Read the model definition and answer for the solid it produces. Units are mm, in the model's axes. Face numbers are marked on the shaded views. A direction names the side the tool comes from. Coordinates: 2 decimals unless noted, no trailing zeros. Order: outer loops, then holes, each group sorted by start corner. A loop starts at its lowest first (then second) coordinate and runs counter-clockwise, first axis right, second up. Notation, with made-up numbers: M 35.25,31.5 L 64.25,31.5 A13 ccw 64.25,43.5 Z; hole C 5.5,62.25 d5. An arc over 180 degrees is marked long. Put each result on its own line as item: value.
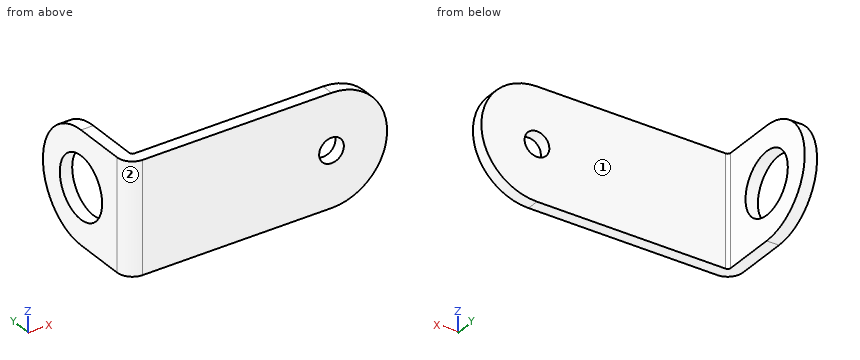
from build123d import *

# Parameters (mm, degrees)
BASE_FLANGE1_DEPTH = 14.2875
SKETCH8_R          = 7.9375
CUT_EXTRUDE3_DEPTH = 72.083846838
SKETCH7_R          = 3.175
CUT_EXTRUDE2_DEPTH = 72.083846838
FILLET1_RADIUS     = 14.2875
FILLET1_LENGTH     = 3.175
FILLET2_RADIUS     = 14.2875
FILLET2_LENGTH     = 3.175


# Sheet-metal steps are written as plain solids
with BuildPart() as part:
    # Sketch1 → Base-Flange1 (new, symmetric)
    with BuildSketch(Plane.XY):
        with BuildLine():
            Line((0, 28.575), (0, 0.7366))
            ThreePointArc((0, 0.7366), (0.215745145, 0.215745145), (0.7366, 0))
            Line((0.7366, 0), (63.5, 0))
            Line((63.5, 0), (63.5, -3.175))
            Line((63.5, -3.175), (0.7366, -3.175))
            ThreePointArc((0.7366, -3.175), (-2.029318885, -2.029318885), (-3.175, 0.7366))
            Line((-3.175, 0.7366), (-3.175, 28.575))
            Line((-3.175, 28.575), (0, 28.575))
        make_face()
    extrude(amount=BASE_FLANGE1_DEPTH, both=True)

    # Sketch8 → Cut-Extrude3 (cut, through all)
    with BuildSketch(Plane(origin=(0, 0, 0), x_dir=(0, 0, -1), z_dir=(1, 0, 0))):
        with Locations(Location((0, 14.2875, 0), (0, 0, 90))):
            Circle(SKETCH8_R)
    extrude(amount=-CUT_EXTRUDE3_DEPTH, mode=Mode.SUBTRACT)

    # Sketch7 → Cut-Extrude2 (cut, through all)
    with BuildSketch(Plane(origin=(0, 0, 0), x_dir=(1, 0, 0), z_dir=(0, 1, 0))):
        with Locations(Location((49.2125, 0, 0), (0, 0, 270))):
            Circle(SKETCH7_R)
    extrude(amount=-CUT_EXTRUDE2_DEPTH, mode=Mode.SUBTRACT)

    # Fillet1: full round fillet: the end face becomes a half cylinder, R = half its width
    fillet1_face = Plane((63.5, -1.5875, 0), x_dir=(0, -1, 0), z_dir=(1, 0, 0))  # on the end face: x along it, z out of the body
    fillet1_slab = fillet1_face.offset(-FILLET1_RADIUS / 2) * Box(FILLET1_LENGTH, 2 * FILLET1_RADIUS, FILLET1_RADIUS, mode=Mode.PRIVATE)  # the body's end, R deep
    fillet1_round = Plane((49.2125, -1.5875, 0), x_dir=(1, 0, 0), z_dir=(0, -1, 0)) * Cylinder(FILLET1_RADIUS, FILLET1_LENGTH, mode=Mode.PRIVATE)  # its axis R under the face
    add(fillet1_slab - fillet1_round, mode=Mode.SUBTRACT)

    # Fillet2: full round fillet: the end face becomes a half cylinder, R = half its width
    fillet2_face = Plane((-1.5875, 28.575, 0), x_dir=(1, 0, 0), z_dir=(0, 1, 0))  # on the end face: x along it, z out of the body
    fillet2_slab = fillet2_face.offset(-FILLET2_RADIUS / 2) * Box(FILLET2_LENGTH, 2 * FILLET2_RADIUS, FILLET2_RADIUS, mode=Mode.PRIVATE)  # the body's end, R deep
    fillet2_round = Plane((-1.5875, 14.2875, 0), x_dir=(0, 1, 0), z_dir=(1, 0, 0)) * Cylinder(FILLET2_RADIUS, FILLET2_LENGTH, mode=Mode.PRIVATE)  # its axis R under the face
    add(fillet2_slab - fillet2_round, mode=Mode.SUBTRACT)


solid = part.part
Q1. Find section C-C on y = 20. Write down the section's boundary in (x, z) (3 decimals).
Answers below:
outline: M -3.175,-13.096 L 0,-13.096 L 0,-5.511 L -3.175,-5.511 Z; M -3.175,5.511 L 0,5.511 L 0,13.096 L -3.175,13.096 Z
Q2. A tool of negligible diameter and unlimited length cuts with its end or side. For the marked faces 1 and 2, from which of +Z, -Z, +X, -X, +Y, -Y can it reach the whole face along a straight path? Write none if from no direction.
Answers below:
face 1: +Z, -Z, +X, +Y
face 2: +Z, -Z, -X, -Y
Q3. Find section B-B on x = 50. Write down the section's boundary in (y, z) (3 decimals).
Answers below:
outline: M -3.175,-14.266 L 0,-14.266 L 0,-3.076 L -3.175,-3.076 Z; M -3.175,3.076 L 0,3.076 L 0,14.266 L -3.175,14.266 Z
Q4. Given pin 1 (7.5 mm diameter, centred on x = 49.21, z = 0, fed in from +Y); pin 2 (1.5 mm diameter, centred on y = 16.5, z = 5, fed in from +X), each flat-ended and moving along its own axis, determine where each tip first touches the part or whether it passes through.
Answers below:
pin 1: stops at y = 0
pin 2: passes through
Q5. Consider line 1 along X through (y, z) = (2, -2.75) (3 decimals); line 2 along X through (y, z) = (-1.45, 0). Determine where each line is inside the solid, lowest interval first.
Answers below:
line 1: x = -3.175 to 0
line 2: x = -2.51 to 46.04, 52.39 to 63.5
Q6. Find section A-A on z = 0. Give the number of separate pieces and of enclosed holes in the cut face, plus the area to 3 significant figures.
Answers below:
separate pieces: 3
enclosed holes: 0
area: 229 mm^2
Q7. Find section D-D on z = -6. Write down the section's boundary in (x, y) (3 decimals), plus the area to 3 significant figures.
Answers below:
outline: M -3.175,0.737 A3.912 ccw 0.737,-3.175 L 62.179,-3.175 L 62.179,0 L 0.737,0 A0.737 cw 0,0.737 L 0,9.091 L -3.175,9.091 Z; M -3.175,19.484 L 0,19.484 L 0,27.254 L -3.175,27.254 Z
area: 258 mm^2
